Can you work these out from the model? Positions are in its coordinate system, mm. Coordinates: 2 decimals unless noted, no trailing zeros. Order: outer loops, then holes, each group sorted by start corner. A loop starts at its lowest first (then second) coordinate and runs counter-clockwise, first axis right, second up. Notation, with made-up numbers: (-7.5, 29.5) -> (21.5, 29.5) arc R8 ccw to (21.5, 36.5) -> close; hole circle Ø8 at (30.5, -2.5). An arc over 180 degrees is marked (long way). Answer in a Markdown table with one row per item. Add a question column.
1. If I drill on line 1 along Y through (x, z) = (-124.5, 1.75); line 2 along Y through (x, z) = (45, 6.5); line 3 along Y through (x, z) = (109, 12), over which ranges is the centre line in solid material (lowest first)? Write a range as [from, to].
2. Imagine slicing it at A-A on x = 45. Write out the boundary of the cut face in (y, z), plus the area to 3 significant figures.
3. Imagine slicing it at B-B on x = -125. Write out the boundary of the cut face in (y, z), plus the area to 3 significant figures.
from build123d import *

# Parameters (mm, degrees)
SKETCH1_W           = 280
SKETCH1_H           = 120
SKETCH1_R           = 3
BOSS_EXTRUDE1_DEPTH = 15
SKETCH2_R           = 5
SKETCH2_R_2         = 1
CUT_EXTRUDE1_DEPTH  = 30


with BuildPart() as part:
    # Sketch1 → Boss-Extrude1 (new body)
    with BuildSketch(Plane.XY):
        Rectangle(SKETCH1_W, SKETCH1_H)
        with Locations((-125, 45)):
            Circle(SKETCH1_R, mode=Mode.SUBTRACT)
        with Locations((125, 45)):
            Circle(SKETCH1_R, mode=Mode.SUBTRACT)
        with Locations((125, -45)):
            Circle(SKETCH1_R, mode=Mode.SUBTRACT)
        with Locations((-125, -45)):
            Circle(SKETCH1_R, mode=Mode.SUBTRACT)
    extrude(amount=BOSS_EXTRUDE1_DEPTH)

    # Sketch2 → Cut-Extrude1 (cut)
    with BuildSketch(Plane.XY.offset(15)):
        with Locations((102, 40)):
            Circle(SKETCH2_R)
        with Locations((45, -20)):
            Circle(SKETCH2_R)
        with Locations((-45, -20)):
            Circle(SKETCH2_R)
        with Locations((-102, 40)):
            Circle(SKETCH2_R)
        with Locations(Location((108.600249206, -43, 0), (0, 0, 180))):
            Circle(SKETCH2_R_2)
        with Locations((94.663331879, -43)):
            Circle(SKETCH2_R_2)
        with Locations((86.854067304, 8.142611191)):
            Circle(SKETCH2_R_2)
        with Locations((66.197255592, -12.527826613)):
            Circle(SKETCH2_R_2)
        with Locations((23.991204862, 6.527590511)):
            Circle(SKETCH2_R_2)
        with Locations((40.954554728, 42.905606098)):
            Circle(SKETCH2_R_2)
        with Locations((-23.997872984, 6.527590511)):
            Circle(SKETCH2_R_2)
        with Locations((-40.96122285, 42.905606098)):
            Circle(SKETCH2_R_2)
        with Locations((-86.860735426, 8.142611191)):
            Circle(SKETCH2_R_2)
        with Locations((-66.203923713, -12.527826613)):
            Circle(SKETCH2_R_2)
        with Locations((-108.606917327, -43)):
            Circle(SKETCH2_R_2)
        with Locations((-94.67, -43)):
            Circle(SKETCH2_R_2)
    extrude(amount=-CUT_EXTRUDE1_DEPTH, mode=Mode.SUBTRACT)


solid = part.part
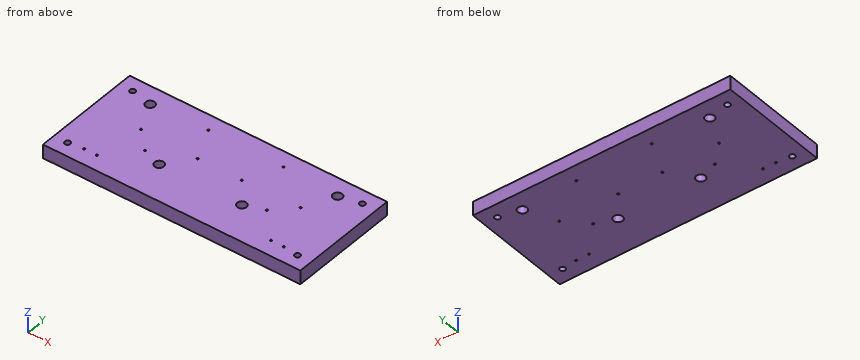
Answers follow:
| question | item | result |
|---|---|---|
| 1 | line 1 | y = [-60, -47.96], [-42.04, 42.04], [47.96, 60] |
| 1 | line 2 | y = [-60, -25], [-15, 60] |
| 1 | line 3 | y = [-60, -43.92], [-42.08, 60] |
| 2 | outline | (-60, 0) -> (-25, 0) -> (-25, 15) -> (-60, 15) -> close; (-15, 0) -> (60, 0) -> (60, 15) -> (-15, 15) -> close |
| 2 | area | 1,650 mm² |
| 3 | outline | (-60, 0) -> (-48, 0) -> (-48, 15) -> (-60, 15) -> close; (-42, 0) -> (42, 0) -> (42, 15) -> (-42, 15) -> close; (48, 0) -> (60, 0) -> (60, 15) -> (48, 15) -> close |
| 3 | area | 1,620 mm² |
